The model under review builds one solid part; all positions refer to its coordinate system, in mm. A direction names the side the tool comes from. Give positions to 0.01 mm unless a question says otherwise; leave off trailing zeros. Order: outer loops, then holes, each group sorted by start corner. A loop starts at its lowest first (then second) coordinate and runs counter-clockwise, first axis right, second up. Notation, with made-up numbers: M 61.25,-15 L 93.25,-15 A26 cw 93.25,21 Z; hole C 54.25,88 d11. An arc over 180 degrees is marked long. One line per question, with ' | ' between items. Start each with the question number.
1. We need section A-A on x = 0. Write out the cut boundary in (y, z), then the cut area to 3 significant figures.
2. Insertion check: P1, Ø3, axis at y = 62.5, z = 48.5, coming from the -X side; P2, Ø3, axis at y = 37.5, z = 33, coming from the +X side; P3, Ø12, axis at x = -40.5, y = 67, coming from the +Z side; P4, Ø7, axis at x = 0, z = -51, coming from the +Y side. Each pin has a flat end and moves straight along its axis. Give the tip position at first contact, or say it passes through.
3. We need section C-C on x = -33. Write out the cut boundary in (y, z), then the cut area to 3 significant figures.
4. We need section D-D on y = 70. Write out the cut boundary in (x, z).
5. Wall thickness on L1, parallel to Z at x = 0, y = 72.75; L2, parallel to X at y = 69, z = 25; L3, parallel to X at y = 68.5, z = -25.5: over which ranges is each line inside the solid? List them lowest first.
6. The part is to be moulded in two halves that separate along Z. For faces 1 (the face through (8.201, 0.986, -62.464)), 2 (the face through (-40, 75, -13)), 3 (the face through (-46.915, 71.056, -25.621)), 4 (the face through (-56.275, 33.031, -17.722)), say which applies: +Z half, -Z half, draft (parallel to the pull), parting line (faces both ways), or undercut.
7. We need section B-B on z = 0. Write out the cut boundary in (x, y), then the cut area to 3 significant figures.
8. For faces 5 (the face through (-14, 67, 39)), 6 (the face through (42.14, 71.06, 23.64)), 7 (the face through (48.408, 37.989, 37.118)), list the 3-axis set-ups (+Z, -Z, +X, -X, +Y, -Y) from which the entire face can be reached by the end or side of a thin tool; tool diameter is ignored.
Autodesk Inventor part; units mm, degrees
ref_plane "Work Plane2" through (0, 10, 0) normal (0, 1, 0) x (1, 0, 0)
ref_plane "YZ Plane" through (0, 0, 0) normal (1, 0, 0) x (0, 1, 0)
ref_plane "XZ Plane" through (0, 0, 0) normal (0, 1, 0) x (-1, 0, 0)
sketch "Sketch1" plane through (0, 0, 0) normal (0, 1, 0) x (-1, 0, 0)
  circle A0 centre (0, 0) radius 63
  circle A1 centre (0, 0) radius 61
  circle A2 centre (0, 0) radius 59
  dimension "Absolute_Diameter" = 126
  dimension "Diameter_No_Outer_Lip" = 122
  dimension "Inner_Cylinder_Diameter" = 118
extrude "Extrusion1" add sketch "Sketch1" along normal blind 2 contours A0
extrude "Extrusion2" add sketch "Sketch1" along normal blind 75 contours A1
sketch "Sketch2" plane through (0, 75, 0) normal (0, 1, 0) x (1, 0, 0)
  circle A0 centre (0, 0) radius 40.5
  circle A1 centre (0, 0) radius 61
  dimension "Lip_Diameter_Out" = 81
  dimension "Top_Outer_Lip_Diameter" = 122
extrude "Extrusion7" add sketch "Sketch2" against normal blind 8
ref_plane "Work Plane2" through (0, 10, 0) normal (0, 1, 0) x (1, 0, 0)
sketch "Sketch3" plane through (0, 10, 0) normal (0, 1, 0) x (1, 0, 0)
  circle A0 centre (0, 0) radius 127.5
  circle A1 centre (-127.5, 0) radius 2.5
  circle A2 centre (-103.1497, -74.9426) radius 2.5
  circle A3 centre (-39.3997, -121.2597) radius 2.5
  circle A4 centre (39.3997, -121.2597) radius 2.5
  circle A5 centre (103.1497, -74.9426) radius 2.5
  circle A6 centre (127.5, 0) radius 2.5
  circle A7 centre (103.1497, 74.9426) radius 2.5
  circle A8 centre (39.3997, 121.2597) radius 2.5
  circle A9 centre (-39.3997, 121.2597) radius 2.5
  circle A10 centre (-103.1497, 74.9426) radius 2.5
  dimension "d27" = 255
  dimension "d28" = 5
  dimension "d31" = 360
extrude "Extrusion8" [suppressed]
sketch "Sketch24" plane through (0, 75, 0) normal (0, 1, 0) x (1, 0, 0)
  circle A0 centre (0, 0) radius 51
  circle A1 centre (0, -51) radius 2.75
  circle A2 centre (44.1673, -25.5) radius 2.75
  circle A3 centre (44.1673, 25.5) radius 2.75
  circle A4 centre (0, 51) radius 2.75
  circle A5 centre (-44.1673, 25.5) radius 2.75
  circle A6 centre (-44.1673, -25.5) radius 2.75
  dimension "d230" = 102
  dimension "d231" = 5.5
  dimension "d234" = 360
extrude "Extrusion30" cut sketch "Sketch24" against normal blind 10 contours A3 A0 | A0 A3 | A2 A0 | A0 A2 | A4 A0 | A0 A4 | A1 A0 | A0 A1 | A5 A0 | A0 A5 | A6 A0 | A0 A6
sketch "Sketch48" plane through (0, 75, 0) normal (0, 1, 0) x (1, 0, 0)
  circle A0 centre (0, 0) radius 51
  dimension "Lip_Height" = 2
  dimension "d897" = 102
properties part number "Cylinder Replacement- 11"
Entries:
1) outline: M 0,-63 L 2,-63 L 2,-61 L 75,-61 L 75,-53.75 L 67,-53.75 L 67,-59 L 0,-59 Z; M 0,59 L 67,59 L 67,53.75 L 75,53.75 L 75,61 L 2,61 L 2,63 L 0,63 Z; M 67,-48.25 L 75,-48.25 L 75,-40.5 L 67,-40.5 Z; M 67,40.5 L 75,40.5 L 75,48.25 L 67,48.25 Z | area: 516 mm^2
2) P1: stops at x = -38.88 | P2: stops at x = 52.24 | P3: stops at z = 50.31 | P4: stops at y = 75
3) outline: M 0,-53.67 L 2,-53.67 L 2,-51.3 L 75,-51.3 L 75,-23.48 L 67,-23.48 L 67,-48.91 L 0,-48.91 Z; M 0,48.91 L 67,48.91 L 67,23.48 L 75,23.48 L 75,51.3 L 2,51.3 L 2,53.67 L 0,53.67 Z | area: 776 mm^2
4) outline: C 0,0 d122; hole C -44.17,-25.5 d5.5; hole C -44.17,25.5 d5.5; hole C 0,0 d81; hole C 0,-51 d5.5; hole C 0,51 d5.5; hole C 44.17,-25.5 d5.5; hole C 44.17,25.5 d5.5
5) L1: z = -61 to -53.75, -48.25 to -40.5, 40.5 to 48.25, 53.75 to 61 | L2: x = -55.64 to -46.87, -41.46 to -31.86, 31.86 to 41.46, 46.87 to 55.64 | L3: x = -55.41 to -46.92, -41.42 to -31.46, 31.46 to 41.42, 46.92 to 55.41
6) face 1: parting line | face 2: draft | face 3: undercut | face 4: undercut
7) outline: M -63,0 L -59,0 L -59,67 L -40.5,67 L -40.5,75 L -61,75 L -61,2 L -63,2 Z; M 40.5,67 L 59,67 L 59,0 L 63,0 L 63,2 L 61,2 L 61,75 L 40.5,75 Z | area: 604 mm^2
8) face 5: -Y | face 6: +Y, -Y | face 7: +Y
